Input: part model. Units: mm. Frame: model coordinates. Face numbers are marked on the shaded views. A direction names the side the tool comes from. Coordinates: 2 decimals unless noted, no trailing zeros. Write each loop counter-clockwise with the first axis right and the second up, starting at its lowest first coordinate (ties: lowest second). Pieces come first, ordered by that corner, then holes. Notation, with made-up numbers: M 87.25,-33 L 98.25,-33 A14 cw 98.25,-8 Z; hole C -23.5,-38 d7. An arc over 180 degrees is marked long. Use CSV: the item, a comma, the result in double quotes.
```python
from build123d import *

# Parameters (mm, degrees)
F0_W     = 1625.6
F0_H     = 482.6
F1_DEPTH = 76.2
F2_W     = 1625.6
F2_H     = 76.2
F3_DEPTH = 914.4
F5_DEPTH = 612.14
F7_DEPTH = 281.94
F8_R     = 50.8
F9_DEPTH = 215.9


with BuildPart() as f1:
    # F0 (on Top) → F1 (new body)
    with BuildSketch(Plane.XY):
        Rectangle(F0_W, F0_H)
    extrude(amount=F1_DEPTH)

    # F2 (on face) → F3 (join)
    with BuildSketch(Plane.XY.offset(76.2)):
        with Locations((0, -203.2)):
            Rectangle(F2_W, F2_H)
    extrude(amount=F3_DEPTH)

    # F4 (on face) → F5 (cut)
    with BuildSketch(Plane(origin=(0, -165.1, 0), x_dir=(-1, 0, 0), z_dir=(0, 1, 0))):
        with BuildLine():
            ThreePointArc((-127, 330.2), (-89.802561, 240.397439), (0, 203.2))
            Line((0, 203.2), (0, 330.2))
            Line((0, 330.2), (-127, 330.2))
        make_face()
        with BuildLine():
            Line((0, 330.2), (0, 203.2))
            ThreePointArc((0, 203.2), (89.802561, 240.397439), (127, 330.2))
            ThreePointArc((127, 330.2), (0, 457.2), (-127, 330.2))
            Line((-127, 330.2), (0, 330.2))
        make_face()
        with BuildLine():
            Line((558.8, 762), (-558.8, 762))
            ThreePointArc((-558.8, 762), (-660.4, 660.4), (-558.8, 558.8))
            Line((-558.8, 558.8), (558.8, 558.8))
            ThreePointArc((558.8, 558.8), (660.4, 660.4), (558.8, 762))
        make_face()
    extrude(amount=-F5_DEPTH, mode=Mode.SUBTRACT)

    # F6 (on face) → F7 (cut)
    with BuildSketch(Plane(origin=(0, -165.1, 0), x_dir=(-1, 0, 0), z_dir=(0, 1, 0))):
        with BuildLine():
            ThreePointArc((736.6, 787.4), (772.521024, 802.278976), (787.4, 838.2))
            Line((787.4, 838.2), (736.6, 838.2))
            Line((736.6, 838.2), (736.6, 787.4))
        make_face()
        with BuildLine():
            Line((736.6, 838.2), (787.4, 838.2))
            ThreePointArc((787.4, 838.2), (700.678976, 874.121024), (736.6, 787.4))
            Line((736.6, 787.4), (736.6, 838.2))
        make_face()
        with BuildLine():
            ThreePointArc((787.4, 177.8), (772.521024, 213.721024), (736.6, 228.6))
            ThreePointArc((736.6, 228.6), (700.678976, 141.878976), (787.4, 177.8))
        make_face()
        with BuildLine():
            ThreePointArc((787.4, 508), (772.521024, 543.921024), (736.6, 558.8))
            Line((736.6, 558.8), (736.6, 508))
            Line((736.6, 508), (736.6, 457.2))
            ThreePointArc((736.6, 457.2), (772.521024, 472.078976), (787.4, 508))
        make_face()
        with BuildLine():
            Line((736.6, 508), (736.6, 558.8))
            ThreePointArc((736.6, 558.8), (685.8, 508), (736.6, 457.2))
            Line((736.6, 457.2), (736.6, 508))
        make_face()
        with BuildLine():
            ThreePointArc((-685.8, 838.2), (-700.678976, 874.121024), (-736.6, 889))
            Line((-736.6, 889), (-736.6, 838.2))
            Line((-736.6, 838.2), (-736.6, 787.4))
            ThreePointArc((-736.6, 787.4), (-700.678976, 802.278976), (-685.8, 838.2))
        make_face()
        with BuildLine():
            ThreePointArc((-685.8, 177.8), (-700.678976, 213.721024), (-736.6, 228.6))
            ThreePointArc((-736.6, 228.6), (-772.521024, 141.878976), (-685.8, 177.8))
        make_face()
        with BuildLine():
            ThreePointArc((-685.8, 508), (-700.678976, 543.921024), (-736.6, 558.8))
            Line((-736.6, 558.8), (-736.6, 508))
            Line((-736.6, 508), (-736.6, 457.2))
            ThreePointArc((-736.6, 457.2), (-700.678976, 472.078976), (-685.8, 508))
        make_face()
        with BuildLine():
            Line((-736.6, 508), (-736.6, 558.8))
            ThreePointArc((-736.6, 558.8), (-787.4, 508), (-736.6, 457.2))
            Line((-736.6, 457.2), (-736.6, 508))
        make_face()
        with BuildLine():
            Line((-736.6, 838.2), (-736.6, 889))
            ThreePointArc((-736.6, 889), (-787.4, 838.2), (-736.6, 787.4))
            Line((-736.6, 787.4), (-736.6, 838.2))
        make_face()
    extrude(amount=-F7_DEPTH, mode=Mode.SUBTRACT)

    # F8 (on face) → F9 (cut)
    with BuildSketch(Plane.XY.offset(76.2)):
        with Locations((-685.8, 114.3)):
            Circle(F8_R)
        with Locations((685.8, 114.3)):
            Circle(F8_R)
    extrude(amount=-F9_DEPTH, mode=Mode.SUBTRACT)


solid = f1.part
```
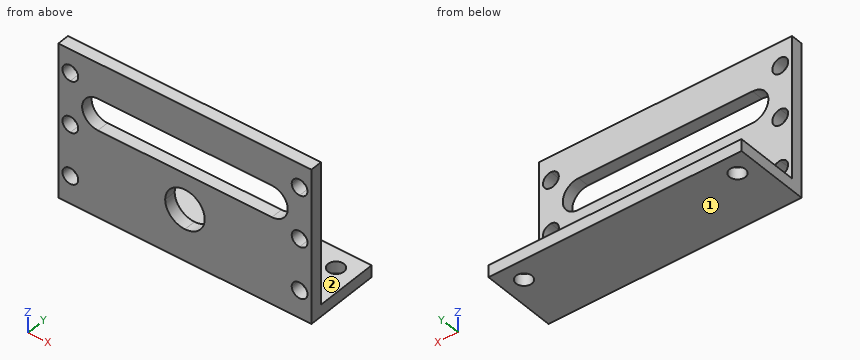
1. Section A-A (x = 408). Return loops of the section in (y, z).
Resolved:
outline,"M -241.3,0 L 241.3,0 L 241.3,76.2 L -165.1,76.2 L -165.1,558.8 L -241.3,558.8 Z; M -241.3,762 L -165.1,762 L -165.1,990.6 L -241.3,990.6 Z"
2. Material intervals for line 1 (X direction, y = -201, z = 838.2); line 2 (Z direction, x = 736.6, y = -190); line 3 (Y direction, x = 497, z = 150.5), sorted ascending. Write a range as [from, to].
Resolved:
line 1,"x = [-812.8, -787.4], [-685.8, 685.8], [787.4, 812.8]"
line 2,"z = [0, 127], [228.6, 457.2], [558.8, 787.4], [889, 990.6]"
line 3,"y = [-241.3, -165.1]"
3. Access query for the marked faces 1 and 2. Directions: +Z, -Z, +X, -X, +Y, -Y. A direction counts if a zero-diameter tool reaches every point of the face in a straight line with its end or side. Return the directions, or none.
Resolved:
face 1,"-Z, +X, -X, +Y, -Y"
face 2,"+Z, +X, -X, +Y"
4. Section C-C (z = 660.4). Return loops of the section in (x, y), then the cut area to 3 significant figures.
Resolved:
outline,"M -812.8,-241.3 L -660.4,-241.3 L -660.4,-165.1 L -812.8,-165.1 Z; M 660.4,-241.3 L 812.8,-241.3 L 812.8,-165.1 L 660.4,-165.1 Z"
area,"23,200 mm^2"
5. Section B-B (y = 114.3). Return loops of the section in (x, z), then the cut area to 3 significant figures.
Resolved:
outline,"M -812.8,0 L -736.6,0 L -736.6,76.2 L -812.8,76.2 Z; M -635,0 L 635,0 L 635,76.2 L -635,76.2 Z; M 736.6,0 L 812.8,0 L 812.8,76.2 L 736.6,76.2 Z"
area,"108,000 mm^2"
6. Section D-D (z = 148). Return loops of the section in (x, y), then the cut area to 3 significant figures.
Resolved:
outline,"M -812.8,-241.3 L -777.74,-241.3 L -777.74,-165.1 L -812.8,-165.1 Z; M -695.46,-241.3 L 695.46,-241.3 L 695.46,-165.1 L -695.46,-165.1 Z; M 777.74,-241.3 L 812.8,-241.3 L 812.8,-165.1 L 777.74,-165.1 Z"
area,"111,000 mm^2"
